from build123d import *

# Parameters (mm, degrees)
BOSS_EXTRUDE1_DEPTH = 15
FILLET1_R           = 10
CUT_EXTRUDE4_REACH  = 30.862
SKETCH7_W           = 7.5
SKETCH7_H           = 10
CUT_EXTRUDE7_REACH  = 30.862
SKETCH10_R          = 1.6
SKETCH9_R           = 1.6
CUT_EXTRUDE8_DEPTH  = 29.861852882
FILLET3_R           = 2
SKETCH3_R           = 2.05
CUT_EXTRUDE9_DEPTH  = 10
SKETCH11_R          = 2.25
CUT_EXTRUDE10_DEPTH = 15


with BuildPart() as part:
    # Sketch2 → Boss-Extrude1 (new body)
    with BuildSketch(Plane.XY):
        with BuildLine():
            Line((-2.5, -6.254565433), (-2.5, -21.254565433))
            Line((-2.5, -21.254565433), (-5, -21.254565433))
            Line((-5, -21.254565433), (-5, -6.254565433))
            Line((-5, -6.254565433), (-5, -5.590169944))
            ThreePointArc((-5, -5.590169944), (0, 7.5), (5, -5.590169944))
            Line((5, -5.590169944), (5, -6.254565433))
            Line((5, -6.254565433), (5, -21.254565433))
            Line((5, -21.254565433), (2.5, -21.254565433))
            Line((2.5, -21.254565433), (2.5, -6.254565433))
            Line((2.5, -6.254565433), (-2.5, -6.254565433))
        make_face()
    extrude(amount=BOSS_EXTRUDE1_DEPTH)

    # Fillet1
    fillet1_edges = [part.edges().sort_by_distance(p)[0] for p in [
        (-5, -5.590169944, 7.5),
        (5, -5.590169944, 7.5),
    ]]
    fillet(fillet1_edges, radius=FILLET1_R)

    # Sketch7 → Cut-Extrude4 (cut, up to next)
    with BuildSketch(Plane(origin=(5, 0, 0), x_dir=(0, 0, -1), z_dir=(1, 0, 0)), mode=Mode.PRIVATE) as cut_extrude4_sk1:
        with Locations((-11.25, -16.254565433)):
            Rectangle(SKETCH7_W, SKETCH7_H)
    cut_extrude4_tool1 = extrude(cut_extrude4_sk1.sketch, amount=-CUT_EXTRUDE4_REACH, mode=Mode.PRIVATE) & part.part
    add(cut_extrude4_tool1.solids().sort_by_distance((5, -16.254565, 11.25))[0], mode=Mode.SUBTRACT)

    # Sketch10 → Cut-Extrude7 (cut, up to next)
    with BuildSketch(Plane.ZY.offset(5), mode=Mode.PRIVATE) as cut_extrude7_sk1:
        with Locations((11.5, -16.254565433)):
            Circle(SKETCH10_R)
    cut_extrude7_tool1 = extrude(cut_extrude7_sk1.sketch, amount=-CUT_EXTRUDE7_REACH, mode=Mode.PRIVATE) & part.part
    add(cut_extrude7_tool1.solids().sort_by_distance((-5, -16.254565, 11.5))[0], mode=Mode.SUBTRACT)

    # Sketch9 → Cut-Extrude8 (cut, through all)
    with BuildSketch(Plane.ZY.offset(5)):
        with Locations((3.5, -16.254565433)):
            Circle(SKETCH9_R)
    extrude(amount=-CUT_EXTRUDE8_DEPTH, mode=Mode.SUBTRACT)

    # Fillet3
    fillet3_edges = [part.edges().sort_by_distance(p)[0] for p in [
        (-2.5, -6.254565433, 7.5),
        (-2.5, -21.254565433, 7.5),
        (2.5, -6.254565433, 7.5),
        (2.5, -21.254565433, 3.75),
        (3.75, -11.254565433, 15),
        (3.75, -11.254565433, 7.5),
    ]]
    fillet(fillet3_edges, radius=FILLET3_R)

    # Sketch3 → Cut-Extrude9 (cut)
    with BuildSketch(Plane(origin=(0, 0, 0), x_dir=(-1, 0, 0), z_dir=(0, 0, -1))):
        Circle(SKETCH3_R)
    extrude(amount=-CUT_EXTRUDE9_DEPTH, mode=Mode.SUBTRACT)

    # Sketch11 → Cut-Extrude10 (cut, symmetric)
    with BuildSketch(Plane.ZY.offset(5)):
        with Locations((7.6, 0)):
            Circle(SKETCH11_R)
    extrude(amount=CUT_EXTRUDE10_DEPTH, both=True, mode=Mode.SUBTRACT)


solid = part.part
Verification items for the finished model (mm, model axes). A direction names the side the tool comes from. Coordinates: 2 decimals unless noted, no trailing zeros. Order: outer loops, then holes, each group sorted by start corner. A loop starts at its lowest first (then second) coordinate and runs counter-clockwise, first axis right, second up. Notation, with made-up numbers: (7.25, 30) -> (61.25, 30) arc R19 ccw to (61.25, 35) -> close; hole circle Ø8 at (20, 13). An arc over 180 degrees is marked (long way). Use CSV: the item, a comma, the result in double quotes. Start each with the question number.
Q1. Section check D-D, the plane x = 0. Record the cut outline in (y, z), and give its area (3 significant figures).
Q2. Section check B-B, the plane z = 11.5. Record the cut outline in (x, y).
Q3. Section check A-A, the plane z = 3.5. Record the cut outline in (x, y), and give its area (3 significant figures).
Q4. Section check C-C, the plane y = 0. Record the cut outline in (x, z), and give its area (3 significant figures).
Q5. Draft check along Z on faces 4 (the cylindrical face through (3.73, -10.65, 14.43)), 5 (the cylindrical face through (-3.768, -15.173, 10.321)), 6 (the flat face through (-2.5, -14, 7)). Enter one of: +Z half, -Z half, draft (parallel to the pull), parting line (faces both ways), or undercut.
Q6. Thickness scan on line 1 along Z through (x, y) = (-4, -16.25); line 2 along Y through (x, z) = (0, 4.25); line 3 along X through (y, z) = (0, 5.25). Record the ranges inside material, lowest first.
Q7. Tool access check on faces 1 (the cylindrical face through (-3.101, -20.684, 7.605)), 2 (the flat face through (4, -11.255, 11)), 3 (the flat face through (5, -14, 6)). Record the directions out of +Z, -Z, +X, -X, +Y, -Y that give a thin tool (end or side, any length) a straight path to the whole face; none if there is none.
Q8. Depth check by flat-ended pin: P1, Ø2, axis at x = 0, y = 0, coming from the -Z side; P2, Ø5, axis at y = -16.25, z = 3.5, coming from the -X side; P3, Ø3, axis at x = -3, y = 3, coming from the -Z side; P4, Ø0.8, axis at x = 3.5, y = -16, coming from the +Z side. Enter the tip coordinate at first touch or a pass-through.
Returned:
1,outline,"(-6.25, 0) -> (-2.05, 0) -> (-2.05, 6.67) arc R2.25 cw to (-2.05, 8.53) -> (-2.05, 10) -> (2.05, 10) -> (2.05, 8.53) arc R2.25 cw to (2.05, 6.67) -> (2.05, 0) -> (7.5, 0) -> (7.5, 15) -> (-6.25, 15) -> close"
1,area,"165 mm^2"
2,outline,"(-6.43, -3.86) arc R10 cw to (-5, -9.01) -> (-5, -14.65) -> (-2.5, -14.65) -> (-2.5, -8.25) arc R2 cw to (-0.5, -6.25) -> (0.5, -6.25) arc R2 cw to (2.5, -8.25) -> (2.5, -11.25) -> (5, -11.25) -> (5, -9.01) arc R10 cw to (6.43, -3.86) arc R7.5 ccw (long way) to start; (-5, -21.25) -> (-4.5, -21.25) arc R2 ccw to (-2.5, -19.25) -> (-2.5, -17.85) -> (-5, -17.85) -> close"
3,outline,"(-6.43, -3.86) arc R10 cw to (-5, -9.01) -> (-5, -14.65) -> (-2.5, -14.65) -> (-2.5, -8.25) arc R2 cw to (-0.5, -6.25) -> (0.5, -6.25) arc R2 cw to (2.5, -8.25) -> (2.5, -14.65) -> (5, -14.65) -> (5, -9.01) arc R10 cw to (6.43, -3.86) arc R7.5 ccw (long way) to start; (-5, -21.25) -> (-4.5, -21.25) arc R2 ccw to (-2.5, -19.25) -> (-2.5, -17.85) -> (-5, -17.85) -> close; (2.5, -19.25) arc R2 ccw to (4.5, -21.25) -> (5, -21.25) -> (5, -17.85) -> (2.5, -17.85) -> close; hole circle Ø4.1 at (0, 0)"
3,area,"218 mm^2"
4,outline,"(-7.5, 0) -> (-2.05, 0) -> (-2.05, 5.35) -> (-7.5, 5.35) -> close; (-7.5, 9.85) -> (-2.05, 9.85) -> (-2.05, 10) -> (2.05, 10) -> (2.05, 9.85) -> (7.5, 9.85) -> (7.5, 15) -> (-7.5, 15) -> close; (2.05, 0) -> (7.5, 0) -> (7.5, 5.35) -> (2.05, 5.35) -> close"
4,area,"135 mm^2"
5,face 4,"+Z half"
5,face 5,"undercut"
5,face 6,"draft"
6,line 1,"z = 0 to 1.9, 5.1 to 9.9, 13.1 to 15"
6,line 2,"y = -6.25 to -2.05, 2.05 to 7.5"
6,line 3,"x = -7.5 to -2.05, 2.05 to 7.5"
7,face 1,"+Z, -Z, -Y"
7,face 2,"+Z, +X, -Y"
7,face 3,"+Z, -Z, +X, -Y"
8,P1,"stops at z = 10"
8,P2,"stops at x = -5"
8,P3,"stops at z = 0"
8,P4,"stops at z = 7.5"
